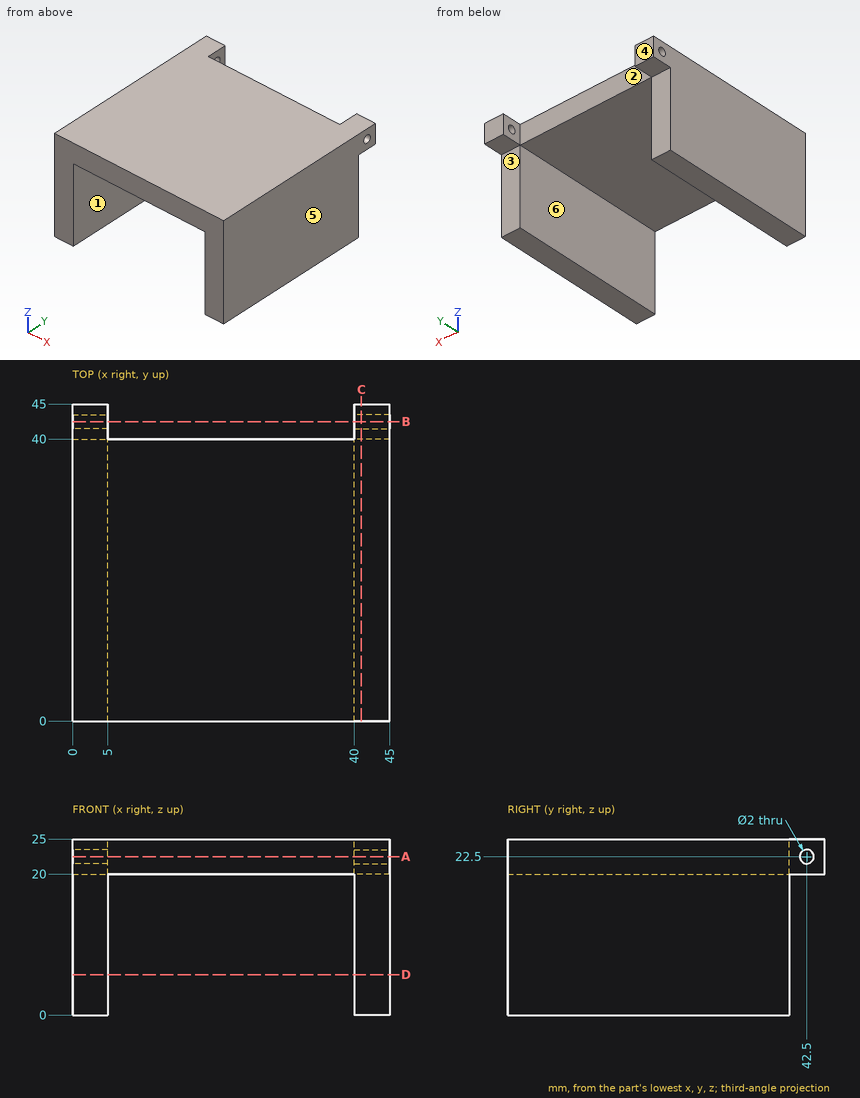
Check sheet for the drawn part. Datum: minimum x, y, z corner. Units: mm. A direction names the side the tool comes from. Round coordinates to 2 decimals unless told otherwise and drop trailing zeros. Order: outer loops, then holes, each group sorted by start corner. A loop starts at its lowest first (then second) coordinate and runs counter-clockwise, first axis right, second up.
(1) Go/stop test with flat-tipped pins: P1, Ø4, axis at x = 20, z = 21.5, coming from the +Y side; P2, Ø1.5, axis at x = 5.5, z = 5, coming from the -Y side; P3, Ø10.5, axis at x = 24.5, y = 27.5, coming from the -Z side. Record where each tip stops, or that it passes through.
(2) Access from +Z, -Z, +X, -X, +Y, -Y to the whole of each face (thin tool, end or side, straight path). Record for the marked faces 1, 2 and 3.
(3) Cross-section at D-D, the plane z = 5.75. Enter the section's corners in (x, y).
(4) Cross-section at C-C, the plane x = 41. Enter the section's corners in (y, z), and give its area (3 significant figures).
(5) Scan lines: probe 1 along X at (y, z) = (2, 9.75); probe 2 along Z at (x, y) = (42.7, 42.5); probe 3 along Z at (x, y) = (21.5, 26). Record each from-to range of solid material in increasing order.
(6) Draft check along X on the marked faces 4, 5 and 6. Enter one of: pulls with the +X half, pulls with the -X half, needs draft (parallel to the pull), parting line crosses it, or undercut.
(7) Cross-section at A-A, the plane z = 22.5. Enter the section's corners in (x, y), and give its area (3 significant figures).
(8) Cross-section at B-B, the plane y = 42.5. Enter the section's corners in (x, z).
Check sheet entries:
1. P1: stops at y = 40
1. P2: stops at y = 0
1. P3: stops at z = 20
2. face 1: -Z, +Y, -Y
2. face 2: +Z, -Z, +Y
2. face 3: -Z, +X, -X, +Y
3. outline: (0, 0) - (5, 0) - (5, 40) - (0, 40) - close; (40, 0) - (45, 0) - (45, 40) - (40, 40) - close
4. outline: (0, 0) - (40, 0) - (40, 20) - (45, 20) - (45, 25) - (0, 25) - close; hole circle Ø2 at (42.5, 22.5)
4. area: 1,020 mm2
5. probe 1: x = 0 to 5, 40 to 45
5. probe 2: z = 20 to 21.5, 23.5 to 25
5. probe 3: z = 20 to 25
6. face 4: needs draft
6. face 5: pulls with the +X half
6. face 6: undercut
7. outline: (0, 0) - (45, 0) - (45, 41.5) - (40, 41.5) - (40, 40) - (5, 40) - (5, 41.5) - (0, 41.5) - close; (0, 43.5) - (5, 43.5) - (5, 45) - (0, 45) - close; (40, 43.5) - (45, 43.5) - (45, 45) - (40, 45) - close
7. area: 1,830 mm2
8. outline: (0, 20) - (5, 20) - (5, 21.5) - (0, 21.5) - close; (0, 23.5) - (5, 23.5) - (5, 25) - (0, 25) - close; (40, 20) - (45, 20) - (45, 21.5) - (40, 21.5) - close; (40, 23.5) - (45, 23.5) - (45, 25) - (40, 25) - close
